Read the model definition and answer for the solid it produces. Units are mm, in the model's axes. A direction names the side the tool comes from. Coordinates: 2 decimals unless noted, no trailing zeros. Write each loop counter-clockwise with the first axis right and the second up, starting at its lowest first coordinate (ties: lowest second). Pieces come first, ordered by that corner, then holes. Notation, with made-up numbers: M 64.25,74 L 120.25,74 A20 cw 120.25,95 Z; hole C 70,-6.75 d2. An arc over 180 degrees is marked long. Write item = value, one per line.
from build123d import *

# Parameters (mm, degrees)
BOSS_EXTRUDE1_DEPTH = 15.7
SKETCH2_R           = 17.25
BOSS_EXTRUDE2_DEPTH = 10
SKETCH4_R           = 0.8
CUT_EXTRUDE1_DEPTH  = 2
SKETCH5_W           = 18.977777778
SKETCH5_H           = 18.977777778
BOSS_EXTRUDE3_DEPTH = 60
SKETCH6_W           = 18.977777778
SKETCH6_H           = 18.977777778
BOSS_EXTRUDE4_DEPTH = 30
CUT_EXTRUDE3_REACH  = 127.825
SKETCH7_R           = 5


with BuildPart() as part:
    # Sketch1 → Boss-Extrude1 (new body)
    with BuildSketch(Plane.XY):
        Polygon((0, 0), (0, -100), (-18.977777778, -100), (-18.977777778, 0), (-15.588888889, 0), (-15.588888889, -16), (-3.388888889, -16), (-3.388888889, 0), align=None)
    extrude(amount=BOSS_EXTRUDE1_DEPTH)

    # Sketch2 → Boss-Extrude2 (add)
    with BuildSketch(Plane.XZ.offset(100)):
        with Locations(Location((-9.488888889, 7.85, 0), (0, 0, 270))):
            Circle(SKETCH2_R)
    extrude(amount=BOSS_EXTRUDE2_DEPTH)

    # Sketch4 → Cut-Extrude1 (cut)
    with BuildSketch(Plane.XZ.offset(110)):
        with Locations(Location((-9.488888889, 7.85, 0), (0, 0, 270))):
            Circle(SKETCH4_R)
    extrude(amount=-CUT_EXTRUDE1_DEPTH, mode=Mode.SUBTRACT)

    # Sketch5 → Boss-Extrude3 (add)
    with BuildSketch(Plane.XY.offset(15.7)):
        with Locations((-9.488888889, -31)):
            Rectangle(SKETCH5_W, SKETCH5_H)
    extrude(amount=BOSS_EXTRUDE3_DEPTH)

    # Sketch6 → Boss-Extrude4 (add)
    with BuildSketch(Plane(origin=(0, -21.511111111, 0), x_dir=(1, 0, 0), z_dir=(0, 1, 0))):
        with Locations((-9.488888889, -55.01587184)):
            Rectangle(SKETCH6_W, SKETCH6_H)
    extrude(amount=BOSS_EXTRUDE4_DEPTH)

    # Sketch7 → Cut-Extrude3 (cut, up to next)
    with BuildSketch(Plane(origin=(0, 0, 45.526982951), x_dir=(-1, 0, 0), z_dir=(0, 0, -1)), mode=Mode.PRIVATE) as cut_extrude3_sk1:
        with Locations((9.488888889, 0.398888889)):
            Circle(SKETCH7_R)
    cut_extrude3_tool1 = extrude(cut_extrude3_sk1.sketch, amount=-CUT_EXTRUDE3_REACH, mode=Mode.PRIVATE) & part.part
    add(cut_extrude3_tool1.solids().sort_by_distance((-9.488889, 0.398889, 45.526983))[0], mode=Mode.SUBTRACT)


solid = part.part
Item 1: For a pull along Z with two mould halves and no side action, classify faces 4 (the face through (-24.793, -104.93, -0.11)), 5 (the face through (-10, -31, 75.7)), 6 (the face through (-10, -40.489, 45)), 7 (the face through (-9, -18, 15.7)) as released by +Z, released by -Z, zero draft, split by the parting line, or undercut.
Worked answers:
face_4 = split by the parting line
face_5 = released by +Z
face_6 = zero draft
face_7 = undercut
Item 2: Flat-ended cylindrical pins translate along their axes: pin 1 (1 mm diameter, centred on x = -12.5, z = 46, fed in from -Y); pin 2 (15 mm diameter, centred on x = -14, y = -13, fed in from +Z); pin 3 (12 mm diameter, centred on x = 2, y = -24.5, fed in from -Z); pin 4 (5 mm diameter, centred on y = -95.5, z = 27, fed in from -X) (3 decimals). Find the tip coordinate at first contact, or state that the pin passes through.
Worked answers:
pin_1 = -40.49
pin_2 = 64.5
pin_3 = 0
pin_4 = through
Item 3: Which of the six approach directions +Z, -Z, +X, -X, +Y, -Y give full straight-line access (tool end or side, diameter ignored) to faces 1 (the face through (0, -33, 29)), 2 (the face through (-2, 0, 8)), 3 (the face through (-9, -100, 16))?
Worked answers:
face_1 = +Z, -Z, +X, +Y
face_2 = -Z, +X, -X, +Y
face_3 = none
Item 4: Find section D-D (y = -93.5). Determine the outline of the cut face in (x, z), and give its area (3 significant figures).
Worked answers:
outline = M -18.98,0 L 0,0 L 0,15.7 L -18.98,15.7 Z
area = 298 mm²
Item 5: Consider line 1 along Z through (x, y) = (-17, -23.5); line 2 along X through (y, z) = (-12.5, 8.5); line 3 along X through (y, z) = (-7, 55). Determine where each line is inside the solid, lowest interval first. Write a range as from..to.
Worked answers:
line_1 = 0..75.7
line_2 = -18.98..-15.59, -3.39..0
line_3 = -18.98..0
Item 6: Find section A-A (x = -6). Determine the outline of the cut face in (y, z), and give its area (3 significant figures).
Worked answers:
outline = M -110,-9.04 L -100,-9.04 L -100,0 L -16,0 L -16,15.7 L -21.51,15.7 L -21.51,45.53 L -3.18,45.53 L -3.18,64.5 L -21.51,64.5 L -21.51,75.7 L -40.49,75.7 L -40.49,15.7 L -100,15.7 L -100,24.74 L -110,24.74 Z; M 3.98,45.53 L 8.49,45.53 L 8.49,64.5 L 3.98,64.5 Z
area = 3,230 mm²
Item 7: Find section B-B (y = -8.5). Determine the outline of the cut face in (x, z).
Worked answers:
outline = M -18.98,0 L -15.59,0 L -15.59,15.7 L -18.98,15.7 Z; M -18.98,45.53 L 0,45.53 L 0,64.5 L -18.98,64.5 Z; M -3.39,0 L 0,0 L 0,15.7 L -3.39,15.7 Z
Item 8: Find section C-C (z = 58). Determine the outline of the cut face in (x, y), and give its area (3 significant figures).
Worked answers:
outline = M -18.98,-40.49 L 0,-40.49 L 0,8.49 L -18.98,8.49 Z; hole C -9.49,0.4 d10
area = 851 mm²
